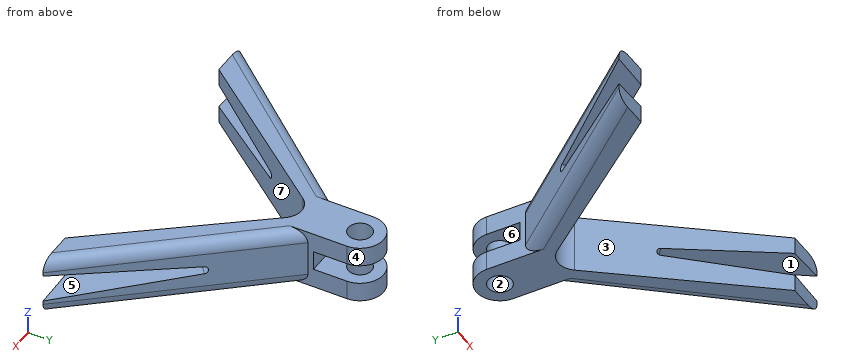
Autodesk Inventor part; units mm, degrees
ref_plane "YZ Plane" through (0, 0, 0) normal (1, 0, 0) x (0, 1, 0)
ref_plane "XZ Plane" through (0, 0, 0) normal (0, 1, 0) x (-1, 0, 0)
ref_plane "XY Plane" through (0, 0, 0) normal (0, 0, 1) x (1, 0, 0)
sketch "Szkic1" plane through (0, 0, 0) normal (0, 0, 1) x (1, 0, 0)
  circle A0 centre (0, 0) radius 3
  arc A1 (6, 0) -> (-6, 0) centre (0, 0) ccw
  line L0 (-6, 0) -> (-6, -10)
  line L1 (6, 0) -> (6, -10)
  line L2 (6, -10) -> (44.5673, -55.9627)
  line L3 (44.5673, -55.9627) -> (34.5673, -55.9627)
  line L4 (34.5673, -55.9627) -> (0, -11.8894)
  line L5 (0, 0) -> (0, -6.4969) construction
  line L6 (-6, 0) -> (-6, -10)
  line L7 (-6, -10) -> (-44.5673, -55.9627)
  line L8 (-44.5673, -55.9627) -> (-34.5673, -55.9627)
  line L9 (-34.5673, -55.9627) -> (0, -11.8894)
  dimension "d0" = 6
  dimension "d1" = 12
  dimension "d2" = 10
  dimension "d3" = 10
  dimension "d4" = 60
  dimension "d5" = 140
  dimension "d6" = 10
extrude "Wyciągnięcie proste1" add sketch "Szkic1" along normal blind 5
sketch "Szkic2" plane through (0, 0, 5) normal (0, 0, 1) x (1, 0, 0)
  circle A0 centre (0, 0) radius 3 construction
  line L0 (-6, 0) -> (-6, -10) construction
  line L1 (-6, -10) -> (-44.5673, -55.9627)
  line L2 (-44.5673, -55.9627) -> (-34.5673, -55.9627)
  line L3 (-34.5673, -55.9627) -> (0, -11.8894)
  line L4 (0, -11.8894) -> (34.5673, -55.9627)
  line L5 (34.5673, -55.9627) -> (44.5673, -55.9627)
  line L6 (44.5673, -55.9627) -> (6, -10)
  line L7 (6, -10) -> (6, 0) construction
  arc A1 (6, 0) -> (-6, 0) centre (0, 0) ccw construction
  line L8 (-6, 0) -> (-6, -10) construction
  line L9 (-6, -8.5404) -> (6, -8.5404)
  line L10 (-6, -10) -> (-6, -8.5404)
  line L11 (6, -10) -> (6, -8.5404)
  line L12 (6, -10) -> (6, 0)
extrude "Wyciągnięcie proste2" add sketch "Szkic2" along normal blind 5
sketch "Szkic3" plane through (0, 0, 10) normal (0, 0, 1) x (1, 0, 0)
  circle A0 centre (0, 0) radius 3
  line L0 (-6, -10) -> (-6, 0)
  arc A1 (6, 0) -> (-6, 0) centre (0, 0) ccw
  line L1 (6, 0) -> (6, -10)
  line L2 (6, -10) -> (44.5673, -55.9627)
  line L3 (44.5673, -55.9627) -> (34.5673, -55.9627)
  line L4 (34.5673, -55.9627) -> (0, -11.8894)
  line L5 (0, -11.8894) -> (-34.5673, -55.9627)
  line L6 (-34.5673, -55.9627) -> (-44.5673, -55.9627)
  line L7 (-44.5673, -55.9627) -> (-6, -10)
extrude "Wyciągnięcie proste3" add sketch "Szkic3" along normal blind 5
sketch "Szkic4" plane through (-44.5673, -55.9627, 0) normal (-0.766, 0.6428, 0) x (0, 0, 1)
  line L0 (0, 0) -> (15, 0)
  line L1 (11.054, 0) -> (7.5, 50.8667)
  line L2 (0, 50.8667) -> (15, 50.8667)
  line L3 (5, 61.1181) -> (10, 61.1181) construction
  line L4 (7.5, 61.1181) -> (7.5, 50.8667) construction
  line L5 (3.946, 0) -> (7.5, 50.8667)
  line L6 (3.946, 0) -> (11.054, 0)
  point P0 (0, 71.5172)
extrude "Wyciągnięcie proste4" cut sketch "Szkic4" against normal blind 25.75
mirror "Odbij1" about plane through (0, 0, 0) normal (1, 0, 0) of "Wyciągnięcie proste4"
fillet "Zaokrąglenie1" radius 5 1 edges at (0, -11.8894, 7.5)
fillet "Zaokrąglenie2" radius 1 1 edges at (9.4991, -18.9866, 7.5)
fillet "Zaokrąglenie3" radius 1 1 edges at (-9.4991, -18.9866, 7.5)
fillet "Zaokrąglenie4" radius 3 4 edges at (-25.2836, -32.9813, 0) (-25.2836, -32.9813, 15) (25.2836, -32.9813, 15) (25.2836, -32.9813, 0)
properties part number "noga"
Geometry check sheet. Reference: the model listing, model coordinates, mm. Face numbers are marked on the shaded views. A direction names the side the tool comes from. Coordinates: 2 decimals unless noted, no trailing zeros. Order: outer loops, then holes, each group sorted by start corner. A loop starts at its lowest first (then second) coordinate and runs counter-clockwise, first axis right, second up. Notation, with made-up numbers: (69, 79) - (100, 79) arc R24 cw to (100, 118) - close; hole circle Ø7 at (20.25, 35.25). An arc over 180 degrees is marked (long way). Answer as a JSON object with one key per item and string values. Group by question number.
Item 1: Scan lines: probe 1 along Y at (x, z) = (0, 12.05); probe 2 along Z at (x, y) = (-0.5, -6); probe 3 along X at (y, z) = (-1, 3.25). Record each from-to range of solid material in increasing order.
Item 2: Draft check along X on the marked faces 1, 2, 3 and 4. Enter one of: +X half, -X half, draft (parallel to the pull), parting line (faces both ways), or undercut.
Item 3: Tool access check on the marked faces 5, 6 and 7. Record the directions out of +Z, -Z, +X, -X, +Y, -Y that give a thin tool (end or side, any length) a straight path to the whole face; none if there is none.
Item 4: Depth check by flat-ended pin: pin 1 Ø8 at (x, y) = (0, 0) entering from -Z; pin 2 Ø5 at (x, z) = (-11.5, 3.5) entering from -Y; pin 3 Ø2 at (y, z) = (-43.5, 11.5) entering from -X; pin 4 Ø5 at (x, z) = (16.5, 11.5) entering from -Y. Enter the tip coordinate at first touch or a pass-through.
Item 5: Sectioned sample at C-C, the plane z = 1.75. Record the cut outline in (x, y).
Item 6: Sectioned sample at A-A, the plane x = 0. Record the cut outline in (y, z).
Item 7: Sectioned sample at B-B, the plane z = 13. Record the cut outline in (x, y).
Resolved:
{
 "1": {"probe 1": "-14.99 to -3, 3 to 6", "probe 2": "0 to 5, 10 to 15", "probe 3": "-6 to -2.83, 2.83 to 6"},
 "2": {"face 1": "+X half", "face 2": "undercut", "face 3": "undercut", "face 4": "parting line"},
 "3": {"face 5": "+X, -Y", "face 6": "+X, -X, +Y", "face 7": "+Z, -Z, -Y"},
 "4": {"pin 1": "z = 0", "pin 2": "y = -29.74", "pin 3": "x = -34.95", "pin 4": "y = -36.11"},
 "5": {"outline": "(-44.21, -55.96) - (-34.57, -55.96) - (-3.93, -16.91) arc R5 cw to (3.93, -16.91) - (34.57, -55.96) - (44.21, -55.96) - (6, -10.42) - (6, 0) arc R6 ccw to (-6, 0) - (-6, -10.42) - close; hole circle Ø6 at (0, 0)"},
 "6": {"outline": "(-14.99, 0) - (-3, 0) - (-3, 5) - (-8.54, 5) - (-8.54, 10) - (-3, 10) - (-3, 15) - (-14.99, 15) - close; (3, 0) - (6, 0) - (6, 5) - (3, 5) - close; (3, 10) - (6, 10) - (6, 15) - (3, 15) - close"},
 "7": {"outline": "(-44.34, -55.96) - (-34.57, -55.96) - (-3.93, -16.91) arc R5 cw to (3.93, -16.91) - (34.57, -55.96) - (44.34, -55.96) - (6, -10.27) - (6, 0) arc R6 ccw to (-6, 0) - (-6, -10.27) - close; hole circle Ø6 at (0, 0)"}
}
